Drawing for the job (mm, zero at the part's lowest x, y, z). A direction names the side the tool comes from. Coordinates: 2 decimals unless noted, no trailing zeros. Write each loop counter-clockwise with the first axis right and the second up, starting at its lowest first coordinate (ties: lowest second). Pieces come first, ordered by that corner, then holes. Notation, with made-up numbers: M -35,72 L -10,72 A14 cw -10,91 Z; hole C 78,29.5 d10. An arc over 180 degrees is marked long. Use CSV: the item, a comma, the result in double quotes. Start each with the question number.
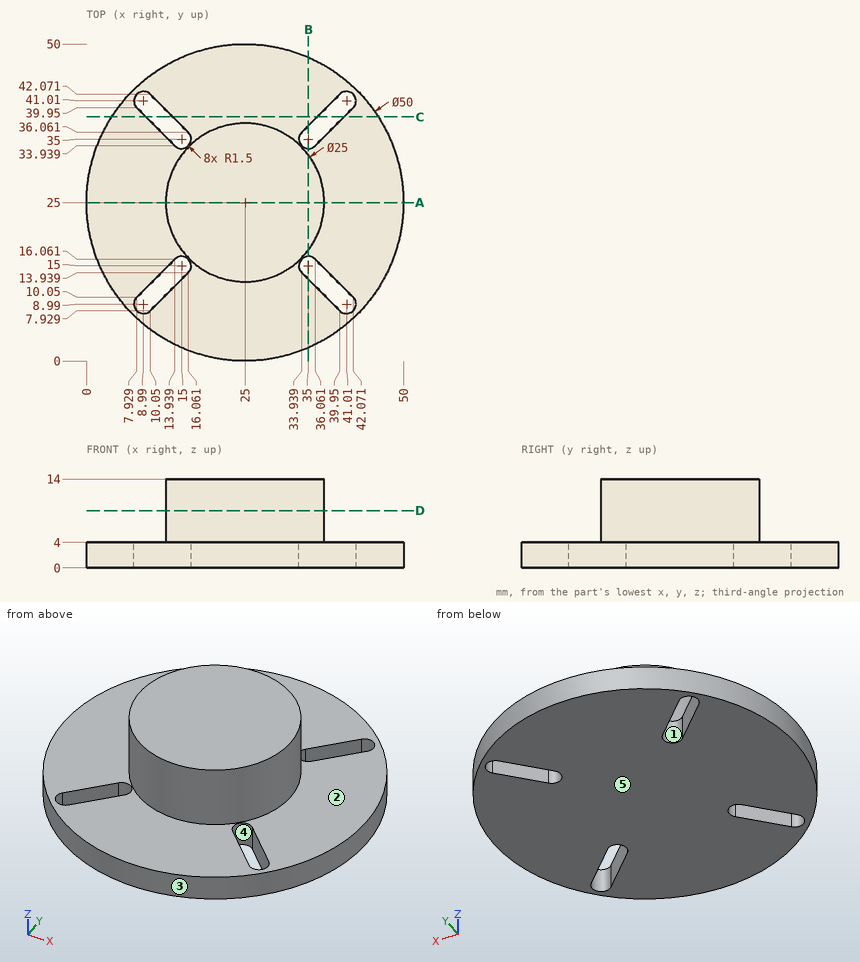
1) Band-saw the part on B-B on x = 35. List the corners of the cut face in (y, z), then the cut area to 3 significant figures.
2) Tool access for the marked faces 1 and 2: list every direction of +Z, -Z, +X, -X, +Y, -Y with a clear straight run to the whole face (end or side of a thin tool).
3) Band-saw the part on A-A on y = 25. List the corners of the cut face in (x, z).
4) Wall check: L1, parallel to X at y = 14, z = 0.5; L2, parallel to Z at x = 46, y = 23; L3, parallel to X at y = 22, z = 12.75 (1 decimal). Give the ranges that are in metal, low to high. Write a range as [from, to].
5) Band-saw the part on D-D on z = 9. List the corners of the cut face in (x, y).
6) Two-plate mould, pull along X, no slides. Class the marked faces 3, 4 and 5: pulls with the +X half, pulls with the -X half, needs draft (parallel to the pull), parting line crosses it, or undercut.
7) Drop flat-ended pins along their axis: P1, Ø4, axis at y = 20, z = 8, coming from the -X side (1 decimal); P2, Ø4, axis at x = 29, y = 42.5, coming from the -Z side; P3, Ø3, axis at x = 26.5, z = 2.5, coming from the +Y side; P4, Ø6, axis at x = 16.5, z = 9.5, coming from the -Y side (1 decimal). Give the stop position or say it passes through.
8) Band-saw the part on C-C on y = 38.5. List the corners of the cut face in (x, z).
Findings below:
1,outline,"M 2.09,0 L 12.88,0 L 12.88,4 L 2.09,4 Z; M 16.5,0 L 33.5,0 L 33.5,4 L 32.5,4 L 32.5,14 L 17.5,14 L 17.5,4 L 16.5,4 Z; M 37.12,0 L 47.91,0 L 47.91,4 L 37.12,4 Z"
1,area,"304 mm2"
2,face 1,"+Z, -Z"
2,face 2,"+Z"
3,outline,"M 0,0 L 50,0 L 50,4 L 37.5,4 L 37.5,14 L 12.5,14 L 12.5,4 L 0,4 Z"
4,L1,"x = [2.55, 11.88], [16.12, 33.88], [38.12, 47.45]"
4,L2,"z = [0, 4]"
4,L3,"x = [12.9, 37.1]"
5,outline,"C 25,25 d25"
6,face 3,"parting line crosses it"
6,face 4,"undercut"
6,face 5,"needs draft"
7,P1,"stops at x = 12.9"
7,P2,"stops at z = 0"
7,P3,"stops at y = 50"
7,P4,"stops at y = 13.8"
8,outline,"M 3.96,0 L 9.38,0 L 9.38,4 L 3.96,4 Z; M 13.62,0 L 36.38,0 L 36.38,4 L 13.62,4 Z; M 40.62,0 L 46.04,0 L 46.04,4 L 40.62,4 Z"
